CAD build for the part. Positions are in the model's coordinates, mm. Coordinates: 2 decimals unless noted, no trailing zeros. Order: outer loops, then holes, each group sorted by start corner. A loop starts at its lowest first (then second) coordinate and runs counter-clockwise, first axis right, second up. Notation, with made-up numbers: (-17, 62) - (15, 62) arc R19 cw to (15, 86) - close; hole circle Ø7 at (26.25, -27). An arc over 180 degrees is marked (long way). Use one line per item in the form item = value.
```python
from build123d import *

# Parameters (mm, degrees)
SKETCH_1_R          = 29.5
SKETCH_1_R_2        = 1.45
EXTRUDE_1_DEPTH     = 5
SKETCH_2_R          = 1.95
CUT_EXTRUDE_1_DEPTH = 62.347371582
FILLET_1_R          = 2


with BuildPart() as part:
    # 草图1 → 凸台-拉伸1 (new body)
    with BuildSketch(Plane(origin=(0, 0, 0), x_dir=(1, 0, 0), z_dir=(0, 1, 0))):
        with BuildLine():
            Line((-36.882678944, 10.135605257), (-47.5, -28.5))
            Line((-47.5, -28.5), (-47.5, -38.5))
            Line((-47.5, -38.5), (47.5, -38.5))
            Line((47.5, -38.5), (47.5, -28.5))
            Line((47.5, -28.5), (36.882678944, 10.135605257))
            ThreePointArc((36.882678944, 10.135605257), (0, 38.25), (-36.882678944, 10.135605257))
        make_face()
        with Locations(Location((0, 0, 0), (0, 0, 270))):
            Circle(SKETCH_1_R, mode=Mode.SUBTRACT)
        with Locations(Location((-34.5, 0, 0), (0, 0, 270))):
            Circle(SKETCH_1_R_2, mode=Mode.SUBTRACT)
        with Locations(Location((-24.395183951, 24.395183951, 0), (0, 0, 270))):
            Circle(SKETCH_1_R_2, mode=Mode.SUBTRACT)
        with Locations(Location((0, 34.5, 0), (0, 0, 270))):
            Circle(SKETCH_1_R_2, mode=Mode.SUBTRACT)
        with Locations(Location((24.395183951, 24.395183951, 0), (0, 0, 270))):
            Circle(SKETCH_1_R_2, mode=Mode.SUBTRACT)
        with Locations(Location((34.5, 0, 0), (0, 0, 270))):
            Circle(SKETCH_1_R_2, mode=Mode.SUBTRACT)
        with Locations(Location((24.395183951, -24.395183951, 0), (0, 0, 270))):
            Circle(SKETCH_1_R_2, mode=Mode.SUBTRACT)
        with Locations(Location((0, -34.5, 0), (0, 0, 270))):
            Circle(SKETCH_1_R_2, mode=Mode.SUBTRACT)
        with Locations(Location((-24.395183951, -24.395183951, 0), (0, 0, 270))):
            Circle(SKETCH_1_R_2, mode=Mode.SUBTRACT)
    extrude(amount=EXTRUDE_1_DEPTH)

    # 草图2 → 切除-拉伸1 (cut, through all)
    with BuildSketch(Plane(origin=(0, 5, 0), x_dir=(1, 0, 0), z_dir=(0, 1, 0))):
        with Locations(Location((-34.5, -33.5, 0), (0, 0, 270))):
            Circle(SKETCH_2_R)
        with Locations(Location((-26.5, -33.5, 0), (0, 0, 270))):
            Circle(SKETCH_2_R)
        with Locations(Location((26.5, -33.5, 0), (0, 0, 270))):
            Circle(SKETCH_2_R)
        with Locations(Location((34.5, -33.5, 0), (0, 0, 270))):
            Circle(SKETCH_2_R)
    extrude(amount=-CUT_EXTRUDE_1_DEPTH, mode=Mode.SUBTRACT)

    # 圆角1
    fillet_1_edges = [part.edges().sort_by_distance(p)[0] for p in [
        (47.5, 2.5, 28.5),
        (47.5, 2.5, 38.5),
        (-47.5, 2.5, 38.5),
        (-47.5, 2.5, 28.5),
    ]]
    fillet(fillet_1_edges, radius=FILLET_1_R)


solid = part.part
```
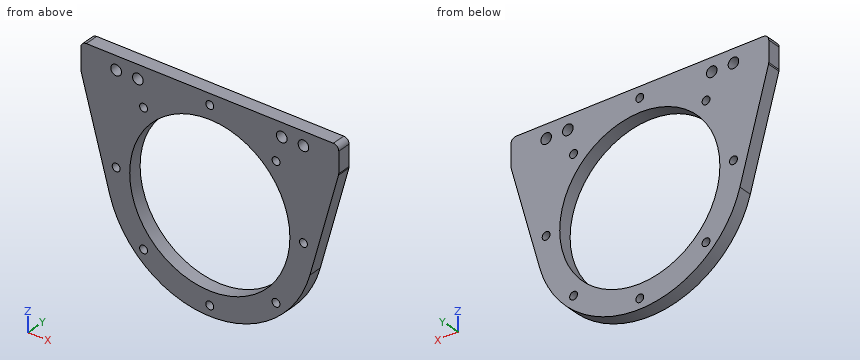
Item 1: Cut at D-D, the plane z = 0. Write the cut outline in (x, y), plus the area to 3 significant figures.
Derived:
outline = (-39.67, 0) - (-35.95, 0) - (-35.95, 5) - (-39.67, 5) - close; (-33.05, 0) - (-29.5, 0) - (-29.5, 5) - (-33.05, 5) - close; (29.5, 0) - (33.05, 0) - (33.05, 5) - (29.5, 5) - close; (35.95, 0) - (39.67, 0) - (39.67, 5) - (35.95, 5) - close
area = 72.7 mm²
Item 2: Cut at B-B, the plane z = 16. Write the cut outline in (x, y), plus the area to 3 significant figures.
Derived:
outline = (-44.06, 0) - (-24.78, 0) - (-24.78, 5) - (-44.06, 5) - close; (24.78, 0) - (44.06, 0) - (44.06, 5) - (24.78, 5) - close
area = 193 mm²
Item 3: Drop a flat-ended pin along its axis: pin 1 (3 mm diameter, centred on x = 35.5, y = 1.5, fed in from -Z). Give the stop position or say it passes through.
Derived:
pin_1 = -17.52
Item 4: Drill centre lines: line 1 (X direction, y = 3.45, z = 1); line 2 (X direction, y = 1.3, z = -21); line 3 (Z direction, x = -1.5, y = 1). Where is each one in solid material? Low to high. Write a range as [from, to].
Derived:
line_1 = [-39.94, -35.55], [-33.45, -29.48], [29.48, 33.45], [35.55, 39.94]
line_2 = [-31.97, -20.72], [20.72, 31.97]
line_3 = [-38.22, -29.46], [29.46, 38.5]
Item 5: Cut at C-C, the plane x = -17. Write the cut outline in (y, z), plus the area to 3 significant figures.
Derived:
outline = (0, -34.26) - (5, -34.26) - (5, -24.11) - (0, -24.11) - close; (0, 24.11) - (5, 24.11) - (5, 38.5) - (0, 38.5) - close
area = 123 mm²
Item 6: Cut at A-A, the plane x = 0. Write the cut outline in (y, z).
Derived:
outline = (0, -38.25) - (5, -38.25) - (5, -35.95) - (0, -35.95) - close; (0, -33.05) - (5, -33.05) - (5, -29.5) - (0, -29.5) - close; (0, 29.5) - (5, 29.5) - (5, 33.05) - (0, 33.05) - close; (0, 35.95) - (5, 35.95) - (5, 38.5) - (0, 38.5) - close
